from build123d import *

# Parameters (mm, degrees)
SKETCH1_W           = 280
SKETCH1_H           = 48.8
BOSS_EXTRUDE1_DEPTH = 4
CUT_EXTRUDE1_DEPTH  = 5
SKETCH3_R           = 7.15
SKETCH3_R_2         = 5.25
BOSS_EXTRUDE2_DEPTH = 8
SKETCH4_R           = 7.15
SKETCH4_R_2         = 2.5
BOSS_EXTRUDE3_DEPTH = 3
SKETCH5_W           = 280
SKETCH5_H           = 48.8
BOSS_EXTRUDE6_DEPTH = 1
SKETCH6_R           = 5.25
CUT_EXTRUDE2_DEPTH  = 1


with BuildPart() as part:
    # Sketch1 → Boss-Extrude1 (new body)
    with BuildSketch(Plane.XY):
        with Locations((18.41484, 11.367285)):
            Rectangle(SKETCH1_W, SKETCH1_H)
    extrude(amount=BOSS_EXTRUDE1_DEPTH)

    # Sketch2 → Cut-Extrude1 (cut, through all)
    with BuildSketch(Plane.XY.offset(4)):
        with BuildLine():
            Line((-1.58516, 23.367285), (-1.58516, 28.617285))
            Line((-1.58516, 28.617285), (3.66484, 28.617285))
            ThreePointArc((3.66484, 28.617285), (-5.297471, 32.329596), (-1.58516, 23.367285))
        make_face()
        with BuildLine():
            Line((3.66484, 28.617285), (-1.58516, 28.617285))
            Line((-1.58516, 28.617285), (-1.58516, 23.367285))
            ThreePointArc((-1.58516, 23.367285), (2.12715, 24.904974), (3.66484, 28.617285))
        make_face()
        with BuildLine():
            ThreePointArc((3.66484, -5.882715), (2.12715, -2.170404), (-1.58516, -0.632715))
            Line((-1.58516, -0.632715), (-1.58516, -5.882715))
            Line((-1.58516, -5.882715), (3.66484, -5.882715))
        make_face()
        with BuildLine():
            Line((-1.58516, -5.882715), (-1.58516, -0.632715))
            ThreePointArc((-1.58516, -0.632715), (-5.297471, -9.595026), (3.66484, -5.882715))
            Line((3.66484, -5.882715), (-1.58516, -5.882715))
        make_face()
        with BuildLine():
            ThreePointArc((43.66484, -5.882715), (42.12715, -2.170404), (38.41484, -0.632715))
            Line((38.41484, -0.632715), (38.41484, -5.882715))
            Line((38.41484, -5.882715), (33.16484, -5.882715))
            ThreePointArc((33.16484, -5.882715), (38.41484, -11.132715), (43.66484, -5.882715))
        make_face()
        with BuildLine():
            Line((38.41484, -5.882715), (38.41484, -0.632715))
            ThreePointArc((38.41484, -0.632715), (34.702529, -2.170404), (33.16484, -5.882715))
            Line((33.16484, -5.882715), (38.41484, -5.882715))
        make_face()
        with BuildLine():
            ThreePointArc((43.66484, 28.617285), (38.41484, 33.867285), (33.16484, 28.617285))
            Line((33.16484, 28.617285), (38.41484, 28.617285))
            Line((38.41484, 28.617285), (38.41484, 23.367285))
            ThreePointArc((38.41484, 23.367285), (42.12715, 24.904974), (43.66484, 28.617285))
        make_face()
        with BuildLine():
            Line((38.41484, 28.617285), (33.16484, 28.617285))
            ThreePointArc((33.16484, 28.617285), (34.702529, 24.904974), (38.41484, 23.367285))
            Line((38.41484, 23.367285), (38.41484, 28.617285))
        make_face()
    extrude(amount=-CUT_EXTRUDE1_DEPTH, mode=Mode.SUBTRACT)

    # Sketch3 → Boss-Extrude2 (add)
    with BuildSketch(Plane.XY.offset(4)):
        with Locations((-1.58516, 28.617285)):
            Circle(SKETCH3_R)
        with Locations((-1.58516, 28.617285)):
            Circle(SKETCH3_R_2, mode=Mode.SUBTRACT)
        with Locations((38.41484, 28.617285)):
            Circle(SKETCH3_R)
        with Locations((38.41484, 28.617285)):
            Circle(SKETCH3_R_2, mode=Mode.SUBTRACT)
        with Locations((-1.58516, -5.882715)):
            Circle(SKETCH3_R)
        with Locations((-1.58516, -5.882715)):
            Circle(SKETCH3_R_2, mode=Mode.SUBTRACT)
        with Locations((38.41484, -5.882715)):
            Circle(SKETCH3_R)
        with Locations((38.41484, -5.882715)):
            Circle(SKETCH3_R_2, mode=Mode.SUBTRACT)
    extrude(amount=BOSS_EXTRUDE2_DEPTH)

    # Sketch4 → Boss-Extrude3 (add)
    with BuildSketch(Plane.XY.offset(12)):
        with Locations((-1.58516, 28.617285)):
            Circle(SKETCH4_R)
        with Locations((-1.58516, 28.617285)):
            Circle(SKETCH4_R_2, mode=Mode.SUBTRACT)
        with Locations((38.41484, 28.617285)):
            Circle(SKETCH4_R)
        with Locations((38.41484, 28.617285)):
            Circle(SKETCH4_R_2, mode=Mode.SUBTRACT)
        with Locations((-1.58516, -5.882715)):
            Circle(SKETCH4_R)
        with Locations((-1.58516, -5.882715)):
            Circle(SKETCH4_R_2, mode=Mode.SUBTRACT)
        with Locations((38.41484, -5.882715)):
            Circle(SKETCH4_R)
        with Locations((38.41484, -5.882715)):
            Circle(SKETCH4_R_2, mode=Mode.SUBTRACT)
    extrude(amount=-BOSS_EXTRUDE3_DEPTH)

    # Sketch5 → Boss-Extrude6 (add)
    with BuildSketch(Plane.XY.offset(4)):
        with Locations((18.41484, 11.367285)):
            Rectangle(SKETCH5_W, SKETCH5_H)
    extrude(amount=BOSS_EXTRUDE6_DEPTH)

    # Sketch6 → Cut-Extrude2 (cut)
    with BuildSketch(Plane(origin=(0, 0, 4), x_dir=(-1, 0, 0), z_dir=(0, 0, -1))):
        with Locations((-38.41484, 28.617285)):
            Circle(SKETCH6_R)
        with Locations((1.58516, 28.617285)):
            Circle(SKETCH6_R)
        with Locations((1.58516, -5.882715)):
            Circle(SKETCH6_R)
        with Locations((-38.41484, -5.882715)):
            Circle(SKETCH6_R)
    extrude(amount=-CUT_EXTRUDE2_DEPTH, mode=Mode.SUBTRACT)


solid = part.part
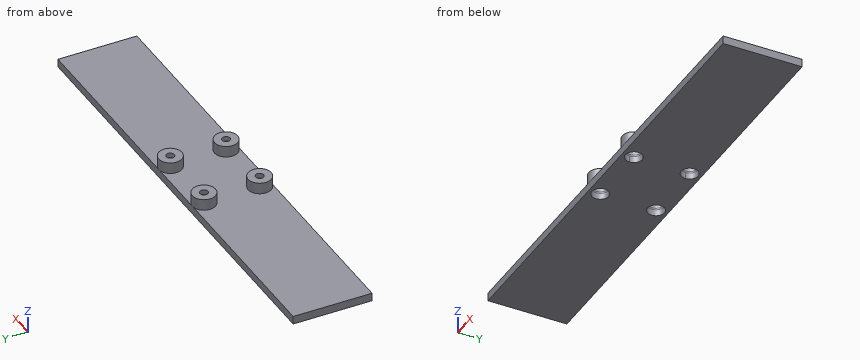
Verification items for the finished model (mm, model axes). Coordinates: 2 decimals unless noted, no trailing zeros. Write each loop counter-clockwise with the first axis right and the second up, starting at its lowest first coordinate (ties: lowest second). Pieces come first, ordered by that corner, then holes. Notation, with made-up numbers: (37, 9) - (50, 9) arc R18 cw to (50, 37) - close; hole circle Ø1 at (-2, -36). An arc over 180 degrees is marked (long way). Answer as a JSON object with one key per item and string values.
(1) Cross-section at C-C on y = 13. Record the cut outline in (x, z), plus the area to 3 significant figures.
Report:
{"outline": "(-121.59, 0) - (158.41, 0) - (158.41, 5) - (-121.59, 5) - close", "area": "1,400 mm^2"}
(2) Gauge pin test, flat ends, axial feed: pin 1 Ø6.5 at (x, y) = (38.41, -5.88) entering from -Z; pin 2 Ø12 at (x, y) = (91.5, 26.5) entering from +Z. Record the tip position at first contact, or that the pin passes through.
Report:
{"pin 1": "z = 9", "pin 2": "z = 5"}
(3) Cross-section at B-B on x = 52. Record the cut outline in (y, z).
Report:
{"outline": "(-13.03, 0) - (35.77, 0) - (35.77, 5) - (-13.03, 5) - close"}
(4) Cross-section at A-A on z = 7. Record the cut outline in (x, y), plus the area to 3 significant figures.
Report:
{"outline": "circle Ø14.3 at (-1.59, -5.88); circle Ø14.3 at (-1.59, 28.62); circle Ø14.3 at (38.41, -5.88); circle Ø14.3 at (38.41, 28.62); hole circle Ø10.5 at (-1.59, -5.88); hole circle Ø10.5 at (-1.59, 28.62); hole circle Ø10.5 at (38.41, -5.88); hole circle Ø10.5 at (38.41, 28.62)", "area": "296 mm^2"}
(5) Thickness scan on line 1 along X through (y, z) = (31.5, 5.25); line 2 along X through (y, z) = (-8, 5.25); line 3 along X through (y, z) = (33, 2.5). Record the ranges inside material, lowest first.
Report:
{"line 1": "-8.13 to -5.97, 2.8 to 4.96, 31.87 to 34.03, 42.8 to 44.96", "line 2": "-8.41 to -6.39, 3.22 to 5.24, 31.59 to 33.61, 43.22 to 45.24", "line 3": "-121.59 to -4.48, 1.31 to 35.52, 41.31 to 158.41"}
